Read the model definition and answer for the solid it produces. Units are mm, in the model's axes. A direction names the side the tool comes from. Give positions to 0.01 mm unless a question says otherwise; leave off trailing zeros. Write each loop counter-clockwise with the first axis right and the second up, starting at its lowest first coordinate (ties: lowest second). Pieces come first, ordered by that corner, then holes. Notation, with made-up numbers: M 58,-35.5 L 97,-35.5 A25 ccw 97,-17.5 Z; hole C 13,37.25 d4. An arc over 180 degrees is marked long. Use a Markdown table: item, result. Add a question column.
Item 1: A cutting plane is placed at A-A on y = 1.75. Determine the outline of the cut face in (x, z), then the cut area to 3 significant figures.
Item 2: The mould has two halves that part along Y. Classify faces 6 (the cylindrical face through (-4.27, 0.03, 10.93)), 7 (the cylindrical face through (17.1, 9.095, 2.535)), 8 (the flat face through (-4, -10.598, 7)): pulls with the +Y half, pulls with the -Y half, needs draft (parallel to the pull), parting line crosses it, or undercut.
Item 3: A cutting plane is placed at B-B on z = 8.25. Determine the outline of the cut face in (x, y), then the cut area to 3 significant figures.
Item 4: Given P1, Ø11.5, axis at x = 4.5, z = 11, coming from the +Y side; P2, Ø2, axis at y = -6, z = 14, coming from the -X side; P3, Ø3.5, axis at x = -11.5, y = 3.5, coming from the +Z side, each flat-ended and moving along its own axis, determine where each tip first touches the part or whether it passes through.
Item 5: For faces 1 (the flat face through (18.526, -2, 2)), 2 (the flat face through (-1.82, 2.6, 9.7)), 3 (the flat face through (5.51, -8.063, 12.148)), 4 (the flat face through (0, 10.598, 4)), 5 (the flat face through (-13, 3, 5)), determine the directions among +Z, -Z, +X, -X, +Y, -Y from which every point of the face is accessible in a straight line to the end or side of a thin tool.
Item 6: Consider probe 1 along Z at (x, y) = (12, 9.75); probe 2 along Y at (x, z) = (6.5, 11.5); probe 3 along Y at (x, z) = (-2.5, 11). Determine where each line is inside the solid, lowest interval first. Write a range as [from, to].
Item 7: A cutting plane is placed at D-D on y = -6. Determine the outline of the cut face in (x, z).
Item 8: A cutting plane is placed at C-C on x = 5.5. Determine the outline of the cut face in (y, z), then the cut area to 3 significant figures.
Autodesk Inventor part; units mm, degrees
ref_plane "YZ Plane" through (0, 0, 0) normal (1, 0, 0) x (0, 1, 0)
ref_plane "XZ Plane" through (0, 0, 0) normal (0, 1, 0) x (-1, 0, 0)
ref_plane "XY Plane" through (0, 0, 0) normal (0, 0, 1) x (1, 0, 0)
sketch "스케치1" plane through (0, 0, 0) normal (0, 0, 1) x (1, 0, 0)
  line L0 (18.5261, -10.5982) -> (-18.5261, -10.5982)
  line L1 (-18.5261, -10.5982) -> (-18.5261, 10.5982)
  line L2 (-18.5261, 10.5982) -> (18.5261, 10.5982)
  line L3 (18.5261, 10.5982) -> (18.5261, -10.5982)
  line L4 (18.5261, -10.5982) -> (-18.5261, 10.5982) construction
  line L5 (-18.5261, -10.5982) -> (18.5261, 10.5982) construction
  point P0 (0, 0)
extrude "돌출1" add sketch "스케치1" along normal blind 5
sketch "스케치2" plane through (0, 0, 5) normal (0, 0, 1) x (1, 0, 0)
  line L0 (-18.5261, -10.5982) -> (18.5261, -10.5982)
  line L1 (-18.5261, 10.5982) -> (-18.5261, -10.5982)
  line L2 (18.5261, -10.5982) -> (-18.5261, -10.5982)
  line L3 (-18.5261, -10.5982) -> (-18.5261, -5.5982)
  line L4 (-18.5261, -5.5982) -> (18.5261, -5.5982)
  line L5 (18.5261, -5.5982) -> (18.5261, -10.5982)
  point P0 (0, 0)
  dimension "d2" = 5
extrude "돌출2" add sketch "스케치2" along normal blind 18.25
sketch "스케치3" plane through (-18.5261, -5.5982, 5) normal (0, 1, 0) x (1, 0, 0)
  line L0 (37.0522, 5) -> (37.0522, -18.25)
  line L1 (37.0522, 0.0749) -> (10.6495, -14.5756)
  line L2 (0, 5) -> (0, 0)
  arc A0 (0, 0) -> (10.6495, -14.5756) centre (23.9382, 6.3119) ccw
  line L3 (37.0522, 0.0749) -> (37.0522, -18.25)
  line L4 (37.0522, -18.25) -> (0, -18.25)
  line L5 (0, -18.25) -> (0, 0)
  point P0 (18.5261, 5)
extrude "돌출3" cut sketch "스케치3" against normal blind 18.25
sketch "스케치4" plane through (0, 0, 5) normal (0, 0, 1) x (1, 0, 0)
  line L0 (-18.5261, -5.5982) -> (18.391, -5.5982)
  line L1 (18.5261, 10.5982) -> (-18.5261, 10.5982)
  line L2 (-1.8195, -5.5982) -> (-6.6451, -5.5982)
  line L3 (-6.6451, -5.5982) -> (-6.6451, 10.5982)
  line L4 (-6.6451, 10.5982) -> (-1.8195, 10.5982)
  line L5 (-1.8195, 10.5982) -> (-1.8195, -5.5982)
  point P0 (0, 0)
extrude "돌출4" add sketch "스케치4" along normal blind 17.25
sketch "스케치5" plane through (-6.6451, -5.5982, 5) normal (-1, 0, 0) x (0, 0, 1)
  arc A0 (9.1518, 0) -> (9.1518, 16.1965) centre (9.1518, 8.0982) ccw
  line L0 (0, 16.1965) -> (17.25, 16.1965)
  line L1 (17.25, 16.1965) -> (17.25, 0)
  circle A1 centre (9.1518, 8.0982) radius 4.0581
  line L2 (14.5756, 0) -> (0, 0)
  line L3 (0, 16.1965) -> (17.25, 16.1965)
  line L4 (9.1518, 16.1965) -> (17.25, 16.1965)
  line L5 (17.25, 16.1965) -> (17.25, 8.0982)
  line L6 (17.25, 0) -> (17.25, 16.1965)
  line L7 (17.25, 0) -> (9.1518, 0)
  line L8 (11.2145, 0) -> (17.25, 0)
  line L9 (17.25, 8.0982) -> (17.25, 0)
  line L10 (17.25, 0) -> (9.1518, 0)
  point P0 (-5, 5.5982)
extrude "돌출5" cut sketch "스케치5" against normal blind 17.25 contours A1
sketch "스케치6" plane through (-1.8195, -5.5982, 5) normal (1, 0, 0) x (0, 0, -1)
  line L0 (-17.25, 16.1965) -> (-17.25, 0)
  line L1 (0, 16.1965) -> (-17.25, 16.1965)
  line L2 (-17.25, 8.0982) -> (-17.25, 16.1965)
  line L3 (-17.25, 16.1965) -> (-8.625, 16.1965)
  line L4 (-17.25, 0) -> (-17.25, 8.0982)
  line L5 (-11.2145, 0) -> (-17.25, 0)
  line L6 (-17.25, 0) -> (-8.3415, 0)
  line L7 (0, 0) -> (-14.5756, 0)
  arc A0 (-17.25, 8.0982) -> (-8.3415, 0) centre (-8.3415, 8.949) ccw
  arc A1 (-8.625, 16.1965) -> (-17.25, 8.0982) centre (-8.625, 7.5543) ccw
  point P0 (5, 5.5982)
extrude "돌출6" cut sketch "스케치6" against normal blind 17.25
fillet "모깎기1" radius 5 2 edges at (-18.5261, 10.5982, 2.5) (18.5261, 10.5982, 2.5)
properties part number "240628_final2"
Filled in:
| question | item | result |
|---|---|---|
| 1 | outline | M -18.53,0 L 18.53,0 L 18.53,5 L -1.82,5 L -1.82,10.16 L -6.65,10.16 L -6.65,5 L -18.53,5 Z; M -6.65,18.14 L -1.82,18.14 L -1.82,22.15 L -6.65,22.15 Z |
| 1 | area | 230 mm² |
| 2 | face 6 | undercut |
| 2 | face 7 | pulls with the +Y half |
| 2 | face 8 | pulls with the -Y half |
| 3 | outline | M -17.42,-10.6 L 12.53,-10.6 L 12.53,-5.6 L -1.82,-5.6 L -1.82,10.6 L -6.65,10.6 L -6.65,-5.6 L -17.42,-5.6 Z |
| 3 | area | 228 mm² |
| 4 | P1 | y = -5.6 |
| 4 | P2 | x = -14.79 |
| 4 | P3 | z = 5 |
| 5 | face 1 | +Z, -Z, +X, +Y, -Y |
| 5 | face 2 | +Z, +X, +Y |
| 5 | face 3 | +Z, +X, -Y |
| 5 | face 4 | +Z, -Z, +X, -X, +Y |
| 5 | face 5 | +Z, -X, +Y |
| 6 | probe 1 | [0, 5] |
| 6 | probe 2 | [-10.6, -5.6] |
| 6 | probe 3 | [-10.6, -0.06], [5.06, 10.6] |
| 7 | outline | M -18.53,0 L 18.53,0 L 18.53,4.93 L -7.88,19.58 A24.76 ccw -18.53,5 Z |
| 8 | outline | M -10.6,0 L 10.6,0 L 10.6,5 L -5.6,5 L -5.6,12.15 L -10.6,12.15 Z |
| 8 | area | 142 mm² |
